```python
from build123d import *

# Parameters (mm, degrees)
F0_W     = 50.8
F0_H     = 203.2
F0_R     = 8.89
F1_DEPTH = 12.7
F3_DEPTH = 2.54
F4_W     = 50.8
F4_H     = 6.35
F5_DEPTH = 25.4
F6_SIZE  = 12.7


with BuildPart() as f1:
    # F0 (on Front) → F1 (new body)
    with BuildSketch(Plane.XZ):
        Rectangle(F0_W, F0_H)
        Circle(F0_R, mode=Mode.SUBTRACT)
    extrude(amount=F1_DEPTH)

    # F2 (on face) → F3 (join)
    with BuildSketch(Plane.XZ.offset(12.7)):
        with BuildLine():
            Line((-13.1982271537, 7.62), (-10.9985226281, 6.35))
            ThreePointArc((-10.9985226281, 6.35), (-10.0755874217, 7.7312701484), (-8.9802561211, 8.9802561211))
            Line((-8.9802561211, 8.9802561211), (-10.7763073453, 10.7763073453))
            ThreePointArc((-10.7763073453, 10.7763073453), (-12.090704906, 9.2775241781), (-13.1982271537, 7.62))
        make_face()
        with BuildLine():
            Line((-15.24, 0), (-12.7, 0))
            ThreePointArc((-12.7, 0), (-12.5913497394, 1.6576826412), (-12.2672579939, 3.2870018728))
            Line((-12.2672579939, 3.2870018728), (-14.7207095926, 3.9444022474))
            ThreePointArc((-14.7207095926, 3.9444022474), (-15.1096196873, 1.9892191694), (-15.24, 0))
        make_face()
        with BuildLine():
            Line((-13.1982271537, -7.62), (-10.9985226281, -6.35))
            ThreePointArc((-10.9985226281, -6.35), (-11.7332700629, -4.860079591), (-12.2672579939, -3.2870018728))
            Line((-12.2672579939, -3.2870018728), (-14.7207095926, -3.9444022474))
            ThreePointArc((-14.7207095926, -3.9444022474), (-14.0799240755, -5.8320955092), (-13.1982271537, -7.62))
        make_face()
        with BuildLine():
            Line((-7.62, -13.1982271537), (-6.35, -10.9985226281))
            ThreePointArc((-6.35, -10.9985226281), (-7.7312701484, -10.0755874217), (-8.9802561211, -8.9802561211))
            Line((-8.9802561211, -8.9802561211), (-10.7763073453, -10.7763073453))
            ThreePointArc((-10.7763073453, -10.7763073453), (-9.2775241781, -12.090704906), (-7.62, -13.1982271537))
        make_face()
        with BuildLine():
            Line((0, -15.24), (0, -12.7))
            ThreePointArc((0, -12.7), (-1.6576826412, -12.5913497394), (-3.2870018728, -12.2672579939))
            Line((-3.2870018728, -12.2672579939), (-3.9444022474, -14.7207095926))
            ThreePointArc((-3.9444022474, -14.7207095926), (-1.9892191694, -15.1096196873), (0, -15.24))
        make_face()
        with BuildLine():
            Line((7.62, -13.1982271537), (6.35, -10.9985226281))
            ThreePointArc((6.35, -10.9985226281), (4.860079591, -11.7332700629), (3.2870018728, -12.2672579939))
            Line((3.2870018728, -12.2672579939), (3.9444022474, -14.7207095926))
            ThreePointArc((3.9444022474, -14.7207095926), (5.8320955092, -14.0799240755), (7.62, -13.1982271537))
        make_face()
        with BuildLine():
            Line((13.1982271537, -7.62), (10.9985226281, -6.35))
            ThreePointArc((10.9985226281, -6.35), (10.0755874217, -7.7312701484), (8.9802561211, -8.9802561211))
            Line((8.9802561211, -8.9802561211), (10.7763073453, -10.7763073453))
            ThreePointArc((10.7763073453, -10.7763073453), (12.090704906, -9.2775241781), (13.1982271537, -7.62))
        make_face()
        with BuildLine():
            Line((15.24, 0), (12.7, 0))
            ThreePointArc((12.7, 0), (12.5913497394, -1.6576826412), (12.2672579939, -3.2870018728))
            Line((12.2672579939, -3.2870018728), (14.7207095926, -3.9444022474))
            ThreePointArc((14.7207095926, -3.9444022474), (15.1096196873, -1.9892191694), (15.24, 0))
        make_face()
        with BuildLine():
            ThreePointArc((10.9985226281, 6.35), (11.7332700629, 4.860079591), (12.2672579939, 3.2870018728))
            Line((12.2672579939, 3.2870018728), (14.7207095926, 3.9444022474))
            ThreePointArc((14.7207095926, 3.9444022474), (14.0799240755, 5.8320955092), (13.1982271537, 7.62))
            Line((13.1982271537, 7.62), (10.9985226281, 6.35))
        make_face()
        with BuildLine():
            Line((7.62, 13.1982271537), (6.35, 10.9985226281))
            ThreePointArc((6.35, 10.9985226281), (7.7312701484, 10.0755874217), (8.9802561211, 8.9802561211))
            Line((8.9802561211, 8.9802561211), (10.7763073453, 10.7763073453))
            ThreePointArc((10.7763073453, 10.7763073453), (9.2775241781, 12.090704906), (7.62, 13.1982271537))
        make_face()
        with BuildLine():
            Line((0, 15.24), (0, 12.7))
            ThreePointArc((0, 12.7), (1.6576826412, 12.5913497394), (3.2870018728, 12.2672579939))
            Line((3.2870018728, 12.2672579939), (3.9444022474, 14.7207095926))
            ThreePointArc((3.9444022474, 14.7207095926), (1.9892191694, 15.1096196873), (0, 15.24))
        make_face()
        with BuildLine():
            Line((-7.62, 13.1982271537), (-6.35, 10.9985226281))
            ThreePointArc((-6.35, 10.9985226281), (-4.860079591, 11.7332700629), (-3.2870018728, 12.2672579939))
            Line((-3.2870018728, 12.2672579939), (-3.9444022474, 14.7207095926))
            ThreePointArc((-3.9444022474, 14.7207095926), (-5.8320955092, 14.0799240755), (-7.62, 13.1982271537))
        make_face()
    extrude(amount=F3_DEPTH)

    # F4 (on face) → F5 (join)
    with BuildSketch(Plane.XZ.offset(12.7)):
        with Locations((0, 98.425)):
            Rectangle(F4_W, F4_H)
        with Locations((0, -98.425)):
            Rectangle(F4_W, F4_H)
    extrude(amount=F5_DEPTH)

    # F6
    f6_edges = [f1.edges().sort_by_distance(p)[0] for p in [
        (-25.4, -38.1, -98.425),
        (25.4, -38.1, -98.425),
        (25.4, -38.1, 98.425),
        (-25.4, -38.1, 98.425),
    ]]
    chamfer(f6_edges, length=F6_SIZE)


solid = f1.part
```
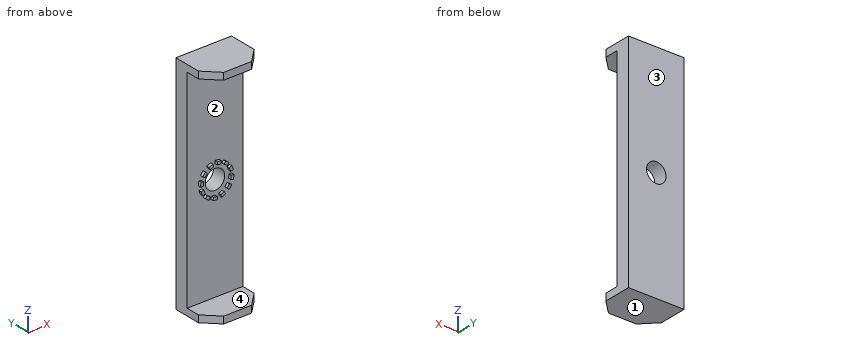
Geometry: final body of the model. Coordinates: model frame, mm. Face numbers are marked on the shaded views. Round coordinates to 2 decimals unless told otherwise and drop trailing zeros. Loops run counter-clockwise (first coordinate to the right, second up) from the corner with the lowest first, then second, coordinate; pieces in that order, holes last. Notation, with made-up numbers: (14.25, 82.25) -> (66.25, 82.25) arc R13 cw to (66.25, 93.25) -> close; hole circle Ø10 at (82, 58.25). An arc over 180 degrees is marked (long way). Use one line per item in the form item = value. Start each with the question number.
1) Draft query along Z for the marked faces 1, 2, 3 and 4. Return one class per face: released by +Z, released by -Z, zero draft, split by the parting line, or undercut.
2) Section A-A on y = -20.5. Output: boundary loops of the cut face in (x, z).
3) First-contact query: P1, Ø1.3, axis at y = -14, z = -14.5, coming from the +X side; P2, Ø2.5, axis at x = 14.5, z = -1, coming from the -Y side; P3, Ø10, axis at x = -18.5, z = -15, coming from the -Y side. Flat tips, straight axial feed; report the tip coordinate or a pass-through.
4) Line query: L1, parallel to Z at x = 0, y = -3.75; L2, parallel to Z at x = 18, y = -24; L3, parallel to Y at x = 7, z = -33. Output: solid intervals per line, ascending.
5) Section D-D on z = 18.5. Output: boundary loops of the cut face in (x, y).
6) Section C-C on y = -30. Output: boundary loops of the cut face in (x, z), then the cut area to 3 significant figures.
7) Section B-B on y = -3. Output: boundary loops of the cut face in (x, z).
Response:
q1.face_1 = released by -Z
q1.face_2 = undercut
q1.face_3 = zero draft
q1.face_4 = undercut
q2.outline = (-25.4, -101.6) -> (25.4, -101.6) -> (25.4, -95.25) -> (-25.4, -95.25) -> close; (-25.4, 95.25) -> (25.4, 95.25) -> (25.4, 101.6) -> (-25.4, 101.6) -> close
q3.P1 = 6.36
q3.P2 = -15.24
q3.P3 = -12.7
q4.L1 = -101.6 to -8.89, 8.89 to 101.6
q4.L2 = -101.6 to -95.25, 95.25 to 101.6
q4.L3 = -12.7 to 0
q5.outline = (-25.4, -12.7) -> (25.4, -12.7) -> (25.4, 0) -> (-25.4, 0) -> close
q6.outline = (-20.8, -101.6) -> (20.8, -101.6) -> (20.8, -95.25) -> (-20.8, -95.25) -> close; (-20.8, 95.25) -> (20.8, 95.25) -> (20.8, 101.6) -> (-20.8, 101.6) -> close
q6.area = 528 mm^2
q7.outline = (-25.4, -101.6) -> (25.4, -101.6) -> (25.4, 101.6) -> (-25.4, 101.6) -> close; hole circle Ø17.78 at (0, 0)
